The listing builds one solid part. Answer for the finished solid, in the listing's coordinates (mm). Coordinates: 2 decimals unless noted, no trailing zeros.
(1) Given P1, Ø1.5, axis at x = 64.5, z = 2, coming from the +Y side; P2, Ø4, axis at x = 43.5, y = 10, coming from the -Z side, each flat-ended and moving along its own axis, determine where each tip first touches the part or whether it passes through.
(2) The part is cut by section A-A on z = 1.75. Give the number of separate pieces and of enclosed holes in the cut face, plus the area to 3 significant figures.
(3) Straight lines are drawn through the part: line 1 (Y direction, x = 82.5, z = 1.8); line 2 (Y direction, x = 29, z = 1.65). For each, find the intervals that lie inside material, in ascending order.
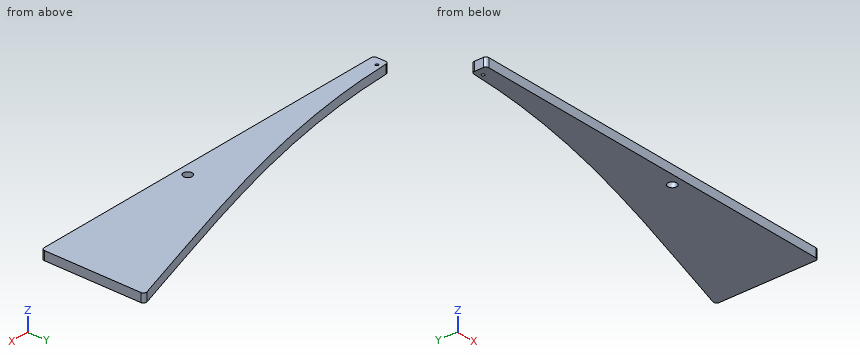
from build123d import *

# Parameters (mm, degrees)
SKETCH_1_R      = 0.5
SKETCH_1_R_2    = 1.5
EXTRUDE_1_DEPTH = 3
FILLET_1_R      = 1


with BuildPart() as part:
    # 草图1 → 凸台-拉伸1 (new body)
    with BuildSketch(Plane.XY):
        with BuildLine():
            Line((-34.1617357, 0), (95.8382643, 0))
            Line((95.8382643, 0), (95.8382643, 35))
            add(Edge.make_bspline(
                [(-34.1617357, 5), (10.689319489, 6.2279178), (53.602553401, 21.947320234), (95.8382643, 35)],
                knots=[0, 0, 0, 0, 1, 1, 1, 1], degree=3))
            Line((-34.1617357, 5), (-34.1617357, 0))
        make_face()
        with Locations((-31.3617357, 3.5)):
            Circle(SKETCH_1_R, mode=Mode.SUBTRACT)
        with Locations((42.6382643, 3.5)):
            Circle(SKETCH_1_R_2, mode=Mode.SUBTRACT)
    extrude(amount=EXTRUDE_1_DEPTH)

    # 圆角1
    fillet_1_edges = [part.edges().sort_by_distance(p)[0] for p in [
        (-34.1617357, 0, 1.5),
        (-34.1617357, 5, 1.5),
        (95.8382643, 35, 1.5),
        (95.8382643, 0, 1.5),
    ]]
    fillet(fillet_1_edges, radius=FILLET_1_R)


solid = part.part
Model answer:
1. P1: stops at y = 25.36
1. P2: stops at z = 0
2. separate pieces: 1
2. enclosed holes: 2
2. area: 2,190 mm2
3. line 1: y = 0 to 30.82
3. line 2: y = 0 to 14.83
